Autodesk Inventor part; units mm, degrees
ref_plane "YZ Plane" through (0, 0, 0) normal (1, 0, 0) x (0, 1, 0)
ref_plane "XZ Plane" through (0, 0, 0) normal (0, 1, 0) x (-1, 0, 0)
ref_plane "XY Plane" through (0, 0, 0) normal (0, 0, 1) x (1, 0, 0)
sketch "Sketch1" plane through (0, 0, 0) normal (0, 0, 1) x (1, 0, 0)
  circle A0 centre (0, 0) radius 31.75
  line L0 (-2.7178, -3.2258) -> (2.7178, -3.2258)
  line L1 (3.2258, -2.7178) -> (3.2258, 2.7178)
  line L2 (2.7178, 3.2258) -> (-2.7178, 3.2258)
  line L3 (-3.2258, 2.7178) -> (-3.2258, -2.7178)
  line L4 (-3.2258, -3.2258) -> (3.2258, 3.2258) construction
  line L5 (3.2258, -3.2258) -> (-3.2258, 3.2258) construction
  arc A1 (-2.7178, 3.2258) -> (-3.2258, 2.7178) centre (-2.7178, 2.7178) ccw
  arc A2 (3.2258, 2.7178) -> (2.7178, 3.2258) centre (2.7178, 2.7178) ccw
  arc A3 (2.7178, -3.2258) -> (3.2258, -2.7178) centre (2.7178, -2.7178) ccw
  arc A4 (-3.2258, -2.7178) -> (-2.7178, -3.2258) centre (-2.7178, -2.7178) ccw
  line L6 (-12.1502, 29.3332) -> (-12.1502, -29.3332) construction
  line L7 (12.1502, 29.3332) -> (12.1502, -29.3332) construction
  line L8 (29.3332, 12.1502) -> (-29.3332, 12.1502) construction
  line L9 (-29.3332, -12.1502) -> (29.3332, -12.1502) construction
  line L10 (12.1502, 29.3332) -> (29.3332, 12.1502) construction
  line L11 (29.3332, 12.1502) -> (29.3332, -12.1502) construction
  line L12 (29.3332, -12.1502) -> (12.1502, -29.3332) construction
  line L13 (12.1502, -29.3332) -> (-12.1502, -29.3332) construction
  line L14 (-12.1502, -29.3332) -> (-29.3332, -12.1502) construction
  line L15 (-29.3332, -12.1502) -> (-29.3332, 12.1502) construction
  line L16 (-29.3332, 12.1502) -> (-12.1502, 29.3332) construction
  line L17 (-12.1502, 29.3332) -> (12.1502, 29.3332) construction
  circle A5 centre (0, 0) radius 35.56
  line L18 (0, 0) -> (13.6082, 32.8532) construction
  line L19 (10.3158, 34.0308) -> (8.8498, 30.4917)
  line L20 (15.3031, 27.8186) -> (16.7691, 31.3578)
  arc A6 (9.6387, 32.3961) -> (10.3158, 34.0308) centre (10.0579, 33.1801) ccw
  arc A7 (16.7691, 31.3578) -> (16.092, 29.7231) centre (16.3499, 30.5739) ccw
  point P0 (16.092, 29.7231)
  dimension "d4" = 63.5
  dimension "d2" = 0.508
  dimension "d3" = 6.4516
  dimension "d9" = 6.985
  dimension "d10" = 3.81
  dimension "d11" = 0.889
extrude "Extrusion1" add sketch "Sketch1" along normal blind 5.08
extrude "Extrusion2" cut sketch "Sketch1" along normal through all contours A0 L19 A6 A5 A7 L20
chamfer "Chamfer2" distance 0.7937 angle 45 4 edges at (9.6387, 32.3961, 2.54) (8.8498, 30.4917, 2.54) (15.3031, 27.8186, 2.54) (16.092, 29.7231, 2.54)
pattern_circular "Circular Pattern1" count 8 over 360 about axis through (0, 0, 0) along (0, 0, 1) of "Extrusion2", "Chamfer2"
properties part number "2in rubberband wheel"
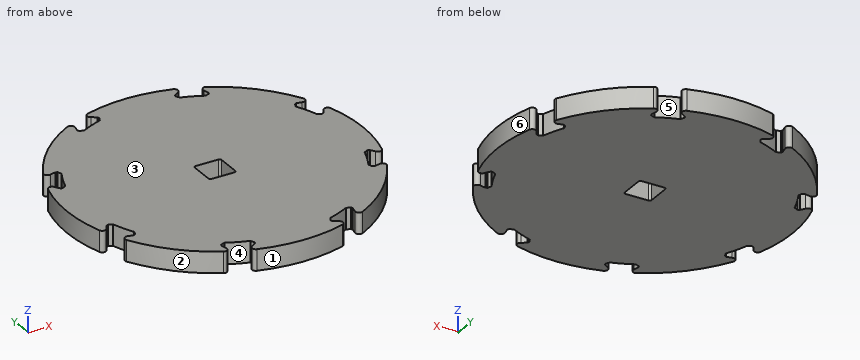
For this review, take the finished solid that the model builds, in its own axes (mm). Face numbers are marked on the shaded views. A direction names the side the tool comes from. Give positions to 0.01 mm unless a question says otherwise; leave off trailing zeros. Loops run counter-clockwise (first coordinate to the right, second up) from the corner with the lowest first, then second, coordinate; pieces in that order, holes last. Notation, with made-up numbers: (43, 44) - (78, 44) arc R19 ccw to (78, 53) - close; hole circle Ø7 at (5.5, -17.5). An arc over 180 degrees is marked (long way). Write each question's results on one line, items separated by ' | '.
(1) Take a section at B-B (x = 22). Give the boundary of the cut face in (y, z), then the cut area to 3 significant figures.
Conclusion:
outline: (-27.94, 0) - (27.94, 0) - (27.94, 5.08) - (-27.94, 5.08) - close | area: 284 mm^2
(2) Take a section at C-C (y = 19.5). Give the boundary of the cut face in (x, z), then the cut area to 3 significant figures.
Conclusion:
outline: (-29.74, 0) - (29.74, 0) - (29.74, 5.08) - (-29.74, 5.08) - close | area: 302 mm^2
(3) Draft analysis for pull direction X (two halves, no side actions). For the marked faces 1, 2, 3 and 4, state which applies: +X half, -X half, draft (parallel to the pull), parting line (faces both ways), or undercut.
Conclusion:
face 1: parting line | face 2: -X half | face 3: draft | face 4: undercut
(4) For pin 1 Ø3 at (x, z) = (-26, 4) entering from +Y; pin 2 Ø3 at (y, z) = (-20, 1.5) entering from +X, all flat-tipped, find the tip position at first contact; note any pin that passes through.
Conclusion:
pin 1: y = 25.77 | pin 2: x = 30.37
(5) Take a section at A-A (y = -1). Give the boundary of the cut face in (x, z).
Conclusion:
outline: (-35.55, 0) - (-3.23, 0) - (-3.23, 5.08) - (-35.55, 5.08) - close; (3.23, 0) - (35.55, 0) - (35.55, 5.08) - (3.23, 5.08) - close
(6) For line 1 along X through (y, z) = (-29, 1.1); line 2 along Y through (x, z) = (-31, 0.75); line 3 along X through (y, z) = (2, 3.45), list the stretches that pass through material, from the lowest coordinate up.
Conclusion:
line 1: -20.58 to -15.79, -12.93 to 12.93, 15.79 to 20.58 | line 2: -17.42 to -15.57, -9.26 to 9.26, 15.57 to 17.42 | line 3: -35.5 to -3.23, 3.23 to 35.5
(7) For the marked faces 5 and 6, list the 3-axis set-ups (+Z, -Z, +X, -X, +Y, -Y) from which the entire face can be reached by the end or side of a thin tool; tool diameter is ignored.
Conclusion:
face 5: +Z, -Z | face 6: +Z, -Z, +X
